Design review of the part built by this model. Coordinates are the model's own, in mm. A direction names the side the tool comes from. Give positions to 0.01 mm unless a question says otherwise; leave off trailing zeros. Loops run counter-clockwise (first coordinate to the right, second up) from the corner with the lowest first, then second, coordinate; pieces in that order, holes last. Notation, with made-up numbers: M -30.5,-7 L -19.5,-7 A26 cw -19.5,32 Z; hole C -38,-5 d5. An arc over 180 degrees is marked long. Use one line per item in the form item = value. Start each with the question number.
from build123d import *

# Parameters (mm, degrees)
BOSS_EXTRUDE1_DEPTH      = 2
SKETCH2_R                = 1
CUT_EXTRUDE1_DEPTH       = 11.827309223
CUT_EXTRUDE2_DEPTH       = 11.827309223
BOSS_EXTRUDE3_DEPTH      = 15
BOSS_EXTRUDE3_DEPTH_BACK = 2
SKETCH4_W                = 13
SKETCH4_H                = 4.75
SKETCH6_W                = 11
SKETCH6_H                = 2
BOSS_EXTRUDE4_DEPTH      = 16
SKETCH7_W                = 11
SKETCH7_H                = 2
BOSS_EXTRUDE5_DEPTH      = 16
SKETCH8_R                = 2
CUT_EXTRUDE3_DEPTH       = 31.850810362
FILLET5_R                = 2
FILLET6_R                = 2
FILLET7_R                = 2
FILLET8_R                = 2
SKETCH10_W               = 2
SKETCH10_H               = 16.939290608
CUT_EXTRUDE4_DEPTH       = 34.719143302
SKETCH11_W               = 13
SKETCH11_H               = 6
CUT_EXTRUDE5_DEPTH       = 28.45564605
SKETCH12_W               = 3
SKETCH12_H               = 2
BOSS_EXTRUDE6_DEPTH      = 3
SKETCH13_W               = 45
SKETCH13_H               = 11
SKETCH13_R               = 2
BOSS_EXTRUDE7_DEPTH      = 3


with BuildPart() as part:
    # Sketch1 → Boss-Extrude1 (new body)
    with BuildSketch(Plane.XY):
        with BuildLine():
            Line((-5.5, -8.425), (5.5, -8.425))
            ThreePointArc((5.5, -8.425), (6.207106781, -8.132106781), (6.5, -7.425))
            Line((6.5, -7.425), (6.5, 7.425))
            ThreePointArc((6.5, 7.425), (6.207106781, 8.132106781), (5.5, 8.425))
            Line((5.5, 8.425), (-5.5, 8.425))
            ThreePointArc((-5.5, 8.425), (-6.207106781, 8.132106781), (-6.5, 7.425))
            Line((-6.5, 7.425), (-6.5, -7.425))
            ThreePointArc((-6.5, -7.425), (-6.207106781, -8.132106781), (-5.5, -8.425))
        make_face()
    extrude(amount=BOSS_EXTRUDE1_DEPTH)

    # Sketch2 → Cut-Extrude1 (cut, through all)
    with BuildSketch(Plane.XY.offset(2)):
        with Locations((0, 6.75)):
            Circle(SKETCH2_R)
        with Locations((0, -2)):
            Circle(SKETCH2_R)
    extrude(amount=-CUT_EXTRUDE1_DEPTH, mode=Mode.SUBTRACT)

    # Sketch3 → Cut-Extrude2 (cut, through all)
    with BuildSketch(Plane.XY.offset(2)):
        with BuildLine():
            Line((1.8, 2.875), (1.8, 1.875))
            ThreePointArc((1.8, 1.875), (0, 0.075), (-1.8, 1.875))
            Line((-1.8, 1.875), (-1.8, 2.875))
            ThreePointArc((-1.8, 2.875), (0, 4.675), (1.8, 2.875))
        make_face()
    extrude(amount=-CUT_EXTRUDE2_DEPTH, mode=Mode.SUBTRACT)

    # Sketch4 → Boss-Extrude3 (add, two sides: drawn at the far end of the back side and taken through both)
    with BuildSketch(Plane(origin=(0, 0, 0), x_dir=(-1, 0, 0), z_dir=(0, 0, -1)).offset(-BOSS_EXTRUDE3_DEPTH_BACK)):
        with Locations((0, -6.05)):
            Rectangle(SKETCH4_W, SKETCH4_H)
    extrude(amount=BOSS_EXTRUDE3_DEPTH + BOSS_EXTRUDE3_DEPTH_BACK)

    # Sketch6 → Boss-Extrude4 (add)
    with BuildSketch(Plane(origin=(6.5, 0, 0), x_dir=(0, 0, -1), z_dir=(1, 0, 0))):
        with Locations((9.5, -7.425)):
            Rectangle(SKETCH6_W, SKETCH6_H)
    extrude(amount=BOSS_EXTRUDE4_DEPTH)

    # Sketch7 → Boss-Extrude5 (add)
    with BuildSketch(Plane.ZY.offset(6.5)):
        with Locations((-9.5, -7.425)):
            Rectangle(SKETCH7_W, SKETCH7_H)
    extrude(amount=BOSS_EXTRUDE5_DEPTH)

    # Sketch8 → Cut-Extrude3 (cut, through all)
    with BuildSketch(Plane(origin=(0, -6.425, 0), x_dir=(1, 0, 0), z_dir=(0, 1, 0))):
        with Locations(Location((15.5, 9.5, 0), (0, 0, 270))):
            Circle(SKETCH8_R)
        with Locations(Location((-15.5, 9.5, 0), (0, 0, 270))):
            Circle(SKETCH8_R)
    extrude(amount=-CUT_EXTRUDE3_DEPTH, mode=Mode.SUBTRACT)

    # Fillet5
    fillet5_edges = [part.edges().sort_by_distance(p)[0] for p in [
        (22.5, -6.425, -9.5),
    ]]
    fillet(fillet5_edges, radius=FILLET5_R - 0.0001)  # a hair under: the kernel refuses the full size

    # Fillet6
    fillet6_edges = [part.edges().sort_by_distance(p)[0] for p in [
        (-22.5, -6.425, -9.5),
    ]]
    fillet(fillet6_edges, radius=FILLET6_R - 0.0001)  # a hair under: the kernel refuses the full size

    # Fillet7
    fillet7_edges = [part.edges().sort_by_distance(p)[0] for p in [
        (6.5, -6.425, -9.5),
    ]]
    fillet(fillet7_edges, radius=FILLET7_R)

    # Fillet8
    fillet8_edges = [part.edges().sort_by_distance(p)[0] for p in [
        (-6.5, -6.425, -9.5),
    ]]
    fillet(fillet8_edges, radius=FILLET8_R)

    # Sketch10 → Cut-Extrude4 (cut, through all)
    with BuildSketch(Plane(origin=(6.5, 0, 0), x_dir=(0, 0, -1), z_dir=(1, 0, 0))):
        with Locations((-1, 4.794645304)):
            Rectangle(SKETCH10_W, SKETCH10_H)
    extrude(amount=-CUT_EXTRUDE4_DEPTH, mode=Mode.SUBTRACT)

    # Sketch11 → Cut-Extrude5 (cut, through all)
    with BuildSketch(Plane(origin=(0, -3.675, 0), x_dir=(1, 0, 0), z_dir=(0, 1, 0))):
        with Locations((0, 1)):
            Rectangle(SKETCH11_W, SKETCH11_H)
    extrude(amount=-CUT_EXTRUDE5_DEPTH, mode=Mode.SUBTRACT)

    # Sketch12 → Boss-Extrude6 (add)
    with BuildSketch(Plane(origin=(0, -3.675, 0), x_dir=(1, 0, 0), z_dir=(0, 1, 0))):
        with Locations((5, 6.2)):
            Rectangle(SKETCH12_W, SKETCH12_H)
    extrude(amount=BOSS_EXTRUDE6_DEPTH)

    # Sketch13 → Boss-Extrude7 (add)
    with BuildSketch(Plane.XZ.offset(8.425)):
        with Locations((0, -9.5)):
            Rectangle(SKETCH13_W, SKETCH13_H)
        with Locations(Location((-15.5, -9.5, 0), (0, 0, 90))):
            Circle(SKETCH13_R, mode=Mode.SUBTRACT)
        with Locations(Location((15.5, -9.5, 0), (0, 0, 90))):
            Circle(SKETCH13_R, mode=Mode.SUBTRACT)
    extrude(amount=BOSS_EXTRUDE7_DEPTH)


solid = part.part
Q1. For faces 4 (the flat face through (5, -2, -5.2)), 5 (the flat face through (-13, -6.425, -10)), 6 (the flat face through (5, -2, -7.2)), 7 (the flat face through (13, -6.425, -9)), 8 (the flat face through (0, -8, -15)), list the 3-axis set-ups (+Z, -Z, +X, -X, +Y, -Y) from which the entire face can be reached by the end or side of a thin tool; tool diameter is ignored.
Q2. Clearance check with flat-ended pins moving along their axes: pin 1 Ø1 at (y, z) = (-6.5, -13.5) entering from +X; pin 2 Ø0.9 at (x, y) = (5, -2.5) entering from -Z; pin 3 Ø5 at (y, z) = (-4.5, -7.5) entering from -X. State where each tip first meets the part, or that it passes through.
Q3. The part is to be moulded in two halves that separate along X. For faces 1 (the cylindrical face through (21.899, -6.995, -9.577)), 2 (the cylindrical face through (-17.483, -8.89, -9.76)), 3 (the flat face through (0, -11.425, -9)), say which applies: pulls with the +X half, pulls with the -X half, needs draft (parallel to the pull), parting line crosses it, or undercut.
Q4. Take a section at B-B on z = -9.5. Give the boundary of the cut face in (x, y) (3 decimals), plus the area to 3 significant figures.
Q5. Wall thickness on probe 1 along X at (y, z) = (-9.55, -9.5); probe 2 along Z at (x, y) = (-15.5, -9.3); probe 3 along X at (y, z) = (-7.7, -9.5): over which ranges is each line inside the solid? List them lowest first.
Q6. Take a section at A-A on x = -15.5. Give the boundary of the cut face in (y, z) (3 decimals), plus the area to 3 significant figures.
Q7. Take a section at C-C on z = -12.5. Give the boundary of the cut face in (x, y) (3 decimals), plus the area to 3 significant figures.
Q8. Take a section at D-D on y = -7.75. Give the boundary of the cut face in (x, z), plus the area to 3 significant figures.
Response values:
q1.face_4 = +Z, +X, -X, +Y
q1.face_5 = +Z, -Z, -X, +Y
q1.face_6 = -Z, +X, -X, +Y
q1.face_7 = +Z, -Z, +X, +Y
q1.face_8 = -Z, +X, -X, +Y, -Y
q2.pin_1 = 21.9
q2.pin_2 = -7.2
q2.pin_3 = -21.9
q3.face_1 = pulls with the +X half
q3.face_2 = undercut
q3.face_3 = needs draft
q4.outline = M -22.5,-11.425 L -17.5,-11.425 L -17.5,-6.425 L -20.5,-6.425 A2 ccw -22.5,-8.425 Z; M -13.5,-11.425 L 13.5,-11.425 L 13.5,-6.425 L 8.5,-6.425 A2 cw 6.5,-4.425 L 6.5,-3.675 L -6.5,-3.675 L -6.5,-4.425 A2 cw -8.5,-6.425 L -13.5,-6.425 Z; M 17.5,-11.425 L 22.5,-11.425 L 22.5,-8.425 A2 ccw 20.5,-6.425 L 17.5,-6.425 Z
q4.area = 221 mm^2
q5.probe_1 = -22.5 to -17.5, -13.5 to 13.5, 17.5 to 22.5
q5.probe_2 = -15 to -11.5, -7.5 to -4
q5.probe_3 = -22.36 to -17.5, -13.5 to 13.5, 17.5 to 22.36
q6.outline = M -11.425,-15 L -6.425,-15 L -6.425,-11.5 L -11.425,-11.5 Z; M -11.425,-7.5 L -6.425,-7.5 L -6.425,-4 L -11.425,-4 Z
q6.area = 35.0 mm^2
q7.outline = M -22.5,-11.425 L 22.5,-11.425 L 22.5,-8.425 A2 ccw 20.5,-6.425 L 8.5,-6.425 A2 cw 6.5,-4.425 L 6.5,-3.675 L -6.5,-3.675 L -6.5,-4.425 A2 cw -8.5,-6.425 L -20.5,-6.425 A2 ccw -22.5,-8.425 Z
q7.area = 261 mm^2
q8.outline = M -22.38,-15 L 22.38,-15 L 22.38,-4 L -22.38,-4 Z; hole C -15.5,-9.5 d4; hole C 15.5,-9.5 d4
q8.area = 467 mm^2
